from build123d import *

# Parameters (mm, degrees)
SKETCH_1_R          = 25
SKETCH_1_R_2        = 3.15
EXTRUDE_1_DEPTH     = 5
SKETCH_2_W          = 9
SKETCH_2_H          = 12.5
CUT_EXTRUDE_3_DEPTH = 6
FILLET_1_R          = 2
SKETCH_3_R          = 8
CUT_EXTRUDE_4_DEPTH = 6


with BuildPart() as part:
    # 草图1 → 凸台-拉伸1 (new body)
    with BuildSketch(Plane(origin=(0, 0, 0), x_dir=(1, 0, 0), z_dir=(0, 1, 0))):
        Circle(SKETCH_1_R)
        with Locations((0, 20)):
            Circle(SKETCH_1_R_2, mode=Mode.SUBTRACT)
        with Locations((17.320508076, 10)):
            Circle(SKETCH_1_R_2, mode=Mode.SUBTRACT)
        with Locations((17.320508076, -10)):
            Circle(SKETCH_1_R_2, mode=Mode.SUBTRACT)
        with Locations((0, -20)):
            Circle(SKETCH_1_R_2, mode=Mode.SUBTRACT)
        with Locations((-17.320508076, -10)):
            Circle(SKETCH_1_R_2, mode=Mode.SUBTRACT)
        with Locations((-17.320508076, 10)):
            Circle(SKETCH_1_R_2, mode=Mode.SUBTRACT)
    extrude(amount=EXTRUDE_1_DEPTH)

    # 草图2 → 切除-拉伸3 (cut, through all)
    with BuildSketch(Plane(origin=(0, 0, 0), x_dir=(1, 0, 0), z_dir=(0, 1, 0))):
        with Locations((-20.5, 0)):
            Rectangle(SKETCH_2_W, SKETCH_2_H)
    extrude(amount=CUT_EXTRUDE_3_DEPTH, mode=Mode.SUBTRACT)

    # 圆角1
    fillet_1_edges = [part.edges().sort_by_distance(p)[0] for p in [
        (-24.206145914, 2.5, -6.25),
        (-24.206145914, 2.5, 6.25),
        (-16, 2.5, -6.25),
        (-16, 2.5, 6.25),
    ]]
    fillet(fillet_1_edges, radius=FILLET_1_R)

    # 草图3 → 切除-拉伸4 (cut, through all)
    with BuildSketch(Plane(origin=(0, 5, 0), x_dir=(1, 0, 0), z_dir=(0, 1, 0))):
        Circle(SKETCH_3_R)
    extrude(amount=-CUT_EXTRUDE_4_DEPTH, mode=Mode.SUBTRACT)


solid = part.part
Build history of the part. All positions in model axes, mm. A direction names the side the tool comes from. Coordinates: 2 decimals unless noted, no trailing zeros. Order: outer loops, then holes, each group sorted by start corner. A loop starts at its lowest first (then second) coordinate and runs counter-clockwise, first axis right, second up. Notation, with made-up numbers: (86, 66.25) - (99, 66.25) arc R32 ccw to (99, 102.25) - close; hole circle Ø9 at (53.5, -15.5). An arc over 180 degrees is marked (long way). Write item = value, one per line. Start each with the question number.
1) Flat gauge pins, fed straight in: pin 1 Ø3 at (x, y) = (-19, 3.5) entering from -Z; pin 2 Ø3 at (x, y) = (-19.5, 3) entering from +Z; pin 3 Ø5.5 at (x, z) = (0, 20) entering from -Y; pin 4 Ø3 at (x, y) = (12.5, 1) entering from -Z. Where does each tip first touch, or does it go through?
2) Saw through at D-D on x = 17.5. Write the cut outline in (y, z).
3) Two-plate mould, pull along X, no slides. Class faces 1 (the face through (-14.3, 2.5, 9.1)), 2 (the face through (-20, 2, 6.25)), 3 (the face through (-16, 2, 0)), 4 (the face through (-14.3, 2.5, -10.9)): pulls with the +X half, pulls with the -X half, needs draft (parallel to the pull), parting line crosses it, or undercut.
4) Wall check: line 1 along Z through (x, y) = (0, 4.4); line 2 along X through (y, z) = (3.65, -9.5); line 3 along X through (y, z) = (2.6, 10). Give the ranges that are in metal, low to high. Write a range as from..to.
5) Saw through at B-B on y = 1.8. Write the cut outline in (x, z).
6) Saw through at C-C on x = 0. Write the cut outline in (y, z), then the cut area to 3 significant figures.
7) Saw through at A-A on z = -20. Write the cut outline in (x, y).
8) 3-axis set-ups, long thin cutter, end or side, ignore diameter. For faces 5 (the face through (6, 5, -6)), 6 (the face through (-20, 2, -6.25)): which of +Z, -Z, +X, -X, +Y, -Y reach the whole face in a straight line?
From the geometry:
q1.pin_1 = -17.85
q1.pin_2 = 17.35
q1.pin_3 = through
q1.pin_4 = -22.45
q2.outline = (0, -17.85) - (5, -17.85) - (5, -13.14) - (0, -13.14) - close; (0, -6.86) - (5, -6.86) - (5, 6.86) - (0, 6.86) - close; (0, 13.14) - (5, 13.14) - (5, 17.85) - (0, 17.85) - close
q3.face_1 = undercut
q3.face_2 = needs draft
q3.face_3 = pulls with the -X half
q3.face_4 = undercut
q4.line_1 = -25..-23.15, -16.85..-8, 8..16.85, 23.15..25
q4.line_2 = -23.12..-20.43, -14.21..14.21, 20.43..23.12
q4.line_3 = -22.91..-20.47, -14.17..14.17, 20.47..22.91
q5.outline = (-23.34, -8.97) arc R25 ccw (long way) to (-23.34, 8.97) arc R2 ccw to (-21.47, 6.25) - (-18, 6.25) arc R2 cw to (-16, 4.25) - (-16, -4.25) arc R2 cw to (-18, -6.25) - (-21.47, -6.25) arc R2 ccw to start; hole circle Ø6.3 at (-17.32, -10); hole circle Ø6.3 at (-17.32, 10); hole circle Ø16 at (0, 0); hole circle Ø6.3 at (0, -20); hole circle Ø6.3 at (0, 20); hole circle Ø6.3 at (17.32, -10); hole circle Ø6.3 at (17.32, 10)
q6.outline = (0, -25) - (5, -25) - (5, -23.15) - (0, -23.15) - close; (0, -16.85) - (5, -16.85) - (5, -8) - (0, -8) - close; (0, 8) - (5, 8) - (5, 16.85) - (0, 16.85) - close; (0, 23.15) - (5, 23.15) - (5, 25) - (0, 25) - close
q6.area = 107 mm^2
q7.outline = (-15, 0) - (-3.15, 0) - (-3.15, 5) - (-15, 5) - close; (3.15, 0) - (15, 0) - (15, 5) - (3.15, 5) - close
q8.face_5 = +Z, -Z, +X, -X, +Y
q8.face_6 = -X, +Y, -Y
